```python
from build123d import *

# Parameters (mm, degrees)
EXTRUDE_THIN3_DEPTH     = 69.85
CUT_EXTRUDE1_DEPTH      = 76.372290574
CUT_EXTRUDE1_DEPTH_BACK = 76.372290574
SKETCH9_R               = 4.064
CUT_EXTRUDE2_DEPTH      = 2.54
LPATTERN1_COUNT         = 2
LPATTERN1_PITCH         = 40.132


# Read off the part's stored shape, not the designer's step: Mirror1
with BuildPart() as part:
    # Sketch6 → Extrude-Thin3 (new body)
    with BuildSketch(Plane.XY):
        Polygon((25.0952, 2.1336), (27.6352, 2.1336), (27.6352, 0), (-27.6352, 0), (-27.6352, 2.1336), (-25.0952, 2.1336), (-25.0952, 2.6416), (-28.1432, 2.6416), (-28.1432, -0.508), (28.1432, -0.508), (28.1432, 2.6416), (25.0952, 2.6416), align=None)
    extrude(amount=EXTRUDE_THIN3_DEPTH)

    # Sketch8 → Cut-Extrude1 (cut, two sides: drawn at the far end of the back side and taken through both)
    with BuildSketch(Plane.XZ.offset(0.508).offset(-CUT_EXTRUDE1_DEPTH_BACK)):
        with BuildLine():
            Line((5, 44.925), (5, 24.925))
            ThreePointArc((5, 24.925), (0, 19.925), (-5, 24.925))
            Line((-5, 24.925), (-5, 44.925))
            ThreePointArc((-5, 44.925), (0, 49.925), (5, 44.925))
        make_face()
    extrude(amount=CUT_EXTRUDE1_DEPTH + CUT_EXTRUDE1_DEPTH_BACK, mode=Mode.SUBTRACT)

    # Sketch9 → Cut-Extrude2 (cut)
    with BuildSketch(Plane.XZ.offset(0.508)):
        with Locations(Location((20.0152, 63.754, 0), (0, 0, 270))):
            Circle(SKETCH9_R)
    cut_extrude2 = extrude(amount=-CUT_EXTRUDE2_DEPTH, mode=Mode.SUBTRACT)

    # Sketch10 → Revolve1 (revolve)
    with BuildSketch(Plane(origin=(0, 0, 63.754), x_dir=(0, -1, 0), z_dir=(0, 0, 1)), mode=Mode.PRIVATE) as revolve1_sk:
        Polygon((0, 24.0792), (1.429807942, 21.6027), (2.016395815, 21.6027), (0, 25.0952), align=None)
    revolve1 = revolve(revolve1_sk.sketch.rotate(Axis((20.0152, 10.109887768, 63.754), (0, -1, 0)), 90), axis=Axis((20.0152, 10.109887768, 63.754), (0, -1, 0)))

    # LPattern1: Cut-Extrude2, Revolve1 ×2
    with Locations(*[(-i * LPATTERN1_PITCH, 0, 0) for i in range(1, LPATTERN1_COUNT)]):
        add(cut_extrude2, mode=Mode.SUBTRACT)
        add(revolve1)

    # Mirror1 outline → Mirror1 (revolve)
    with BuildSketch(Plane(origin=(20.0152, 0, 6.096), x_dir=(1, 0, 0), z_dir=(0, 0, 1))):
        Polygon((3.18411819, -0.508), (1.5875, -1.429807942), (1.5875, -2.016395815), (4.20011819, -0.508), align=None)
    revolve(axis=Axis((20.0152, 0, 6.096), (0, 1, 0)))

    # Mirror1 2 outline → Mirror1 2 (revolve)
    with BuildSketch(Plane(origin=(-20.1168, 0, 6.096), x_dir=(1, 0, 0), z_dir=(0, 0, 1))):
        Polygon((3.18411819, -0.508), (1.5875, -1.429807942), (1.5875, -2.016395815), (4.20011819, -0.508), align=None)
    revolve(axis=Axis((-20.1168, 0, 6.096), (0, 1, 0)))

    # Mirror1 3 outline → Mirror1 3 (revolve, cut)
    with BuildSketch(Plane(origin=(20.0152, 0, 6.096), x_dir=(1, 0, 0), z_dir=(0, 0, 1))):
        Polygon((3.18411819, -0.508), (4.064, 0), (0, 0), (0, -0.508), align=None)
    revolve(axis=Axis((20.0152, 0, 6.096), (0, 1, 0)), mode=Mode.SUBTRACT)

    # Mirror1 4 outline → Mirror1 4 (revolve, cut)
    with BuildSketch(Plane(origin=(-20.1168, 0, 6.096), x_dir=(1, 0, 0), z_dir=(0, 0, 1))):
        Polygon((3.18411819, -0.508), (4.064, 0), (0, 0), (0, -0.508), align=None)
    revolve(axis=Axis((-20.1168, 0, 6.096), (0, 1, 0)), mode=Mode.SUBTRACT)


solid = part.part
```
Design review of the part built by this model. Coordinates are the model's own, in mm. A direction names the side the tool comes from. Coordinates: 2 decimals unless noted, no trailing zeros. Order: outer loops, then holes, each group sorted by start corner. A loop starts at its lowest first (then second) coordinate and runs counter-clockwise, first axis right, second up. Notation, with made-up numbers: (71.5, 35.5) - (84.5, 35.5) arc R17 cw to (84.5, 57.5) - close; hole circle Ø1 at (20, 19.5). An arc over 180 degrees is marked (long way). Answer in a Markdown table with one row per item.
(1) Clearance check with flat-ended pins moving along their axes: pin 1 (2 mm diameter, centred on x = -14.5, z = 15.5, fed in from +Y); pin 2 (1.9 mm diameter, centred on x = -20.12, z = 63.75, fed in from -Y); pin 3 (1.3 mm diameter, centred on x = 27, z = 36.5, fed in from -Y); pin 4 (3.5 mm diameter, centred on x = -20.12, z = 6.1, fed in from -Y). State where each tip first meets the part, or that it passes through.
Checked values:
| item | result |
|---|---|
| pin 1 | y = 0 |
| pin 2 | through |
| pin 3 | y = -0.51 |
| pin 4 | y = -2.02 |
(2) Consider section A-A on x = 0. State the section outline as (y, z) points (3 decimals), plus the area to 3 significant figures.
Checked values:
| item | result |
|---|---|
| outline | (-0.508, 0) - (0, 0) - (0, 19.925) - (-0.508, 19.925) - close; (-0.508, 49.925) - (0, 49.925) - (0, 69.85) - (-0.508, 69.85) - close |
| area | 20.2 mm^2 |
(3) For faces 1 (the flat face through (-7, -0.508, 34)), 2 (the cylindrical face through (0.11, -0.25, 19.926)), 3 (the flat face through (-27.635, 1, 34)), list the 3-axis set-ups (+Z, -Z, +X, -X, +Y, -Y) from which the entire face can be reached by the end or side of a thin tool; tool diameter is ignored.
Checked values:
| item | result |
|---|---|
| face 1 | -Y |
| face 2 | +Y, -Y |
| face 3 | +Z, -Z |
(4) Consider section B-B on z = 21. State the section outline as (x, y) points, plus the area to 3 significant figures.
Checked values:
| item | result |
|---|---|
| outline | (-28.14, -0.51) - (-3.1, -0.51) - (-3.1, 0) - (-27.64, 0) - (-27.64, 2.13) - (-25.1, 2.13) - (-25.1, 2.64) - (-28.14, 2.64) - close; (3.1, -0.51) - (28.14, -0.51) - (28.14, 2.64) - (25.1, 2.64) - (25.1, 2.13) - (27.64, 2.13) - (27.64, 0) - (3.1, 0) - close |
| area | 30.7 mm^2 |
(5) The part is to be moulded in two halves that separate along X. For faces 4 (the flat face through (-28.143, 1, 34)), 5 (the conical face through (21.633, -1.922, 6.767)), 6 (the cylindrical face through (18.85, -1.73, 5.02)), 7 (the flat face through (-0.1, -0.2, 69.85)), say which applies: released by +X, released by -X, zero draft, split by the parting line, or undercut.
Checked values:
| item | result |
|---|---|
| face 4 | released by -X |
| face 5 | undercut |
| face 6 | undercut |
| face 7 | zero draft |
(6) Wall thickness on line 1 along Y through (x, z) = (26, 19); line 2 along X through (y, z) = (-0.3, 7); line 3 along X through (y, z) = (1, 55): over which ranges is each line inside the solid? List them lowest first. Write a range as from..to.
Checked values:
| item | result |
|---|---|
| line 1 | -0.51..0, 2.13..2.64 |
| line 2 | -28.14..-23.54, -16.69..16.59, 23.44..28.14 |
| line 3 | -28.14..-27.64, 27.64..28.14 |
(7) Consider section D-D on x = -6.5. State the section outline as (y, z) points, plus the area to 3 significant figures.
Checked values:
| item | result |
|---|---|
| outline | (-0.51, 0) - (0, 0) - (0, 69.85) - (-0.51, 69.85) - close |
| area | 35.5 mm^2 |
(8) Consider section C-C on z = 12.5. State the section outline as (x, y) points, plus the area to 3 significant figures.
Checked values:
| item | result |
|---|---|
| outline | (-28.14, -0.51) - (28.14, -0.51) - (28.14, 2.64) - (25.1, 2.64) - (25.1, 2.13) - (27.64, 2.13) - (27.64, 0) - (-27.64, 0) - (-27.64, 2.13) - (-25.1, 2.13) - (-25.1, 2.64) - (-28.14, 2.64) - close |
| area | 33.9 mm^2 |
